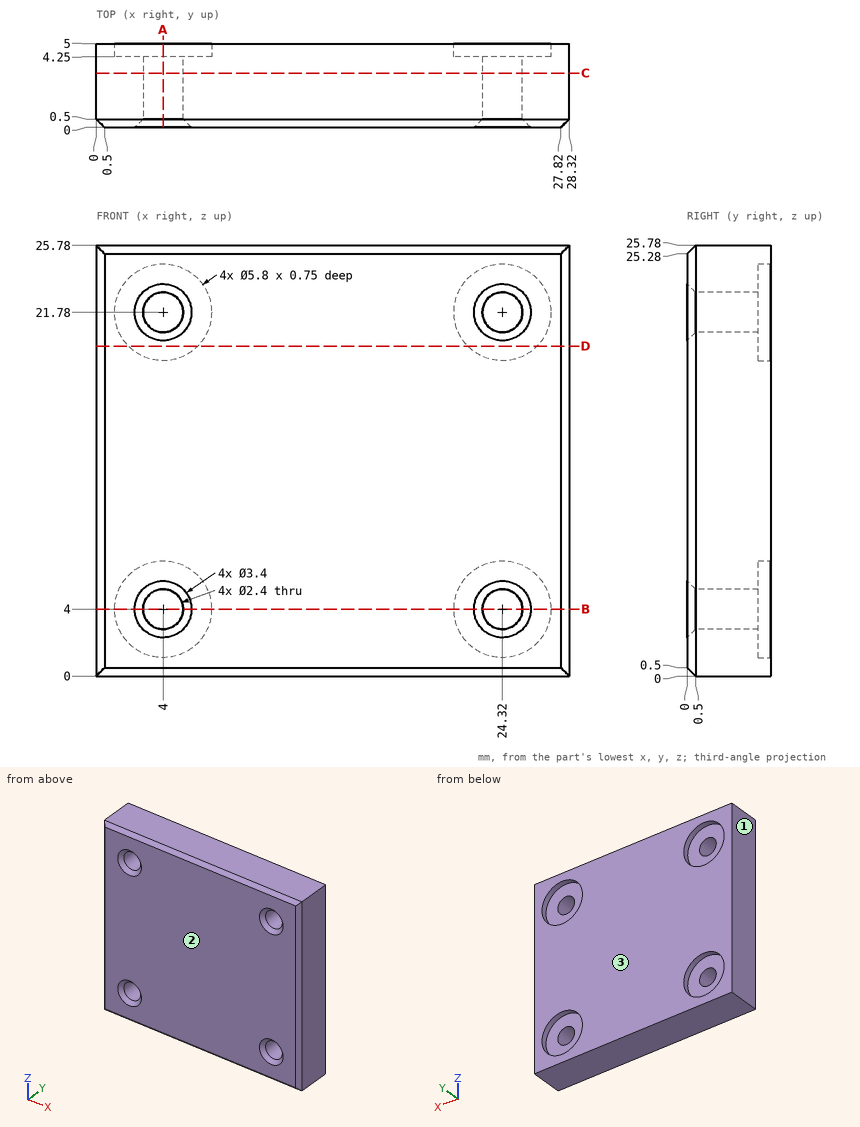
Drawing for the job (mm, zero at the part's lowest x, y, z). Round coordinates to 2 decimals unless told otherwise and drop trailing zeros. Write each loop counter-clockwise with the first axis right and the second up, starting at its lowest first coordinate (ties: lowest second). Pieces come first, ordered by that corner, then holes. Notation, with made-up numbers: M 14.5,-33 L 21.5,-33 A34 cw 21.5,6 Z; hole C 41.5,41 d7. An arc over 180 degrees is marked long. Put each result on its own line as item: value.
Item 1: Cut at D-D (z = 19.75). List the corners of the cut face in (x, y).
Responses:
outline: M 0,0.5 L 0.5,0 L 27.82,0 L 28.32,0.5 L 28.32,5 L 26.39,5 L 26.39,4.25 L 22.25,4.25 L 22.25,5 L 6.07,5 L 6.07,4.25 L 1.93,4.25 L 1.93,5 L 0,5 Z
Item 2: Flat gauge pins, fed straight in: P1, Ø5, axis at x = 24.32, z = 21.78, coming from the +Y side; P2, Ø1.4, axis at x = 4, z = 4, coming from the -Y side. Where does each tip first touch, or does it go through?
Responses:
P1: y = 4.25
P2: through
Item 3: Cut at A-A (x = 4). List the corners of the cut face in (y, z), and give its area (4 significant figures).
Responses:
outline: M 0,0.5 L 0.5,0 L 5,0 L 5,1.1 L 4.25,1.1 L 4.25,2.8 L 0.5,2.8 L 0,2.3 Z; M 0,5.7 L 0.5,5.2 L 4.25,5.2 L 4.25,6.9 L 5,6.9 L 5,18.88 L 4.25,18.88 L 4.25,20.58 L 0.5,20.58 L 0,20.08 Z; M 0,23.48 L 0.5,22.98 L 4.25,22.98 L 4.25,24.68 L 5,24.68 L 5,25.78 L 0.5,25.78 L 0,25.28 Z
area: 99.05 mm²
Item 4: Cut at C-C (y = 3.25). List the corners of the cut face in (x, z).
Responses:
outline: M 0,0 L 28.32,0 L 28.32,25.78 L 0,25.78 Z; hole C 4,4 d2.4; hole C 4,21.78 d2.4; hole C 24.32,4 d2.4; hole C 24.32,21.78 d2.4
Item 5: Cut at B-B (z = 4). List the corners of the cut face in (x, y).
Responses:
outline: M 0,0.5 L 0.5,0 L 2.3,0 L 2.8,0.5 L 2.8,4.25 L 1.1,4.25 L 1.1,5 L 0,5 Z; M 5.2,0.5 L 5.7,0 L 22.62,0 L 23.12,0.5 L 23.12,4.25 L 21.42,4.25 L 21.42,5 L 6.9,5 L 6.9,4.25 L 5.2,4.25 Z; M 25.52,0.5 L 26.02,0 L 27.82,0 L 28.32,0.5 L 28.32,5 L 27.22,5 L 27.22,4.25 L 25.52,4.25 Z
Item 6: Probe L1, parallel to Z at x = 4, y = 4.7; L2, parallel to X at y = 1.9, z = 4; L3, parallel to Z at x = 24.32, y = 2.8. List the from-to ranges inside material, lowest first. Write a range as from..to.
Responses:
L1: 0..1.1, 6.9..18.88, 24.68..25.78
L2: 0..2.8, 5.2..23.12, 25.52..28.32
L3: 0..2.8, 5.2..20.58, 22.98..25.78
Item 7: Mould opens along Y. For the marked faces 1, 2 and 3 say: +Y half, -Y half, draft (parallel to the pull), parting line (faces both ways), or undercut.
Responses:
face 1: draft
face 2: -Y half
face 3: +Y half
